from build123d import *

# Parameters (mm, degrees)
F0_W     = 31.75
F0_H     = 50.8
F0_W_2   = 3.175
F0_H_2   = 12.7
F0_W_3   = 12.7
F0_H_3   = 3.175
F0_W_4   = 19.05
F0_H_4   = 38.1
F1_DEPTH = 3.175


# Not quite as in the source:
# - a feature names something its author has since deleted; it is built from what else it names


with BuildPart() as f1:
    # F0 (on Top) → F1 (new body)
    with BuildSketch(Plane.XY):
        with Locations((-8.6727611423, -50.1471598029)):
            Rectangle(F0_W, F0_H)
        with Locations((-40.4227611423, -50.1471598029)):
            Rectangle(F0_W, F0_H)
        Polygon((-81.6977611423, 51.4528401971), (-88.0477611423, 51.4528401971), (-88.0477611423, 45.1028401971), (-84.8727611423, 45.1028401971), (-84.8727611423, 32.4028401971), (-84.8727611423, 19.7028401971), (-84.8727611423, 7.0028401971), (-84.8727611423, -5.6971598029), (-84.8727611423, -18.3971598029), (-88.0477611423, -18.3971598029), (-88.0477611423, -24.7471598029), (-68.9977611423, -24.7471598029), (-56.2977611423, -24.7471598029), (-24.5477611423, -24.7471598029), (7.2022388577, -24.7471598029), (19.9022388577, -24.7471598029), (38.9522388577, -24.7471598029), (38.9522388577, -18.3971598029), (35.7772388577, -18.3971598029), (35.7772388577, -5.6971598029), (35.7772388577, 7.0028401971), (35.7772388577, 19.7028401971), (35.7772388577, 32.4028401971), (35.7772388577, 45.1028401971), (38.9522388577, 45.1028401971), (38.9522388577, 51.4528401971), (32.6022388577, 51.4528401971), (32.6022388577, 48.2778401971), (19.9022388577, 48.2778401971), (7.2022388577, 48.2778401971), (-5.4977611423, 48.2778401971), (-18.1977611423, 48.2778401971), (-30.8977611423, 48.2778401971), (-43.5977611423, 48.2778401971), (-56.2977611423, 48.2778401971), (-68.9977611423, 48.2778401971), (-81.6977611423, 48.2778401971), align=None)
        with Locations((-86.4602611423, 26.0528401971)):
            Rectangle(F0_W_2, F0_H_2)
        with Locations((-86.4602611423, 0.6528401971)):
            Rectangle(F0_W_2, F0_H_2)
        with Locations((37.3647388577, 0.6528401971)):
            Rectangle(F0_W_2, F0_H_2)
        with Locations((37.3647388577, 26.0528401971)):
            Rectangle(F0_W_2, F0_H_2)
        with Locations((-62.6477611423, 49.8653401971)):
            Rectangle(F0_W_3, F0_H_3)
        with Locations((-11.8477611423, 49.8653401971)):
            Rectangle(F0_W_3, F0_H_3)
        with Locations((-37.2477611423, 49.8653401971)):
            Rectangle(F0_W_3, F0_H_3)
        with Locations((-78.5227611423, -43.7971598029)):
            Rectangle(F0_W_4, F0_H_4)
        with Locations((29.4272388577, -43.7971598029)):
            Rectangle(F0_W_4, F0_H_4)
        with Locations((13.5522388577, 49.8653401971)):
            Rectangle(F0_W_3, F0_H_3)
    extrude(amount=F1_DEPTH)


solid = f1.part
The model under review builds one solid part; all positions refer to its coordinate system, in mm. A direction names the side the tool comes from. Coordinates: 2 decimals unless noted, no trailing zeros. Write each loop counter-clockwise with the first axis right and the second up, starting at its lowest first coordinate (ties: lowest second). Pieces come first, ordered by that corner, then holes. Notation, with made-up numbers: (-3, 85) -> (4, 85) arc R27 cw to (4, 101) -> close; hole circle Ø6 at (-36, -1.75). An arc over 180 degrees is marked (long way). Answer in a Markdown table with one row per item.
1. For faces 4 (the flat face through (-63, -24.747, 2)), 5 (the flat face through (37, -5.697, 2)), 6 (the flat face through (-68.998, 50, 2)), list the 3-axis set-ups (+Z, -Z, +X, -X, +Y, -Y) from which the entire face can be reached by the end or side of a thin tool; tool diameter is ignored.
Answers below:
| item | result |
|---|---|
| face 4 | +Z, -Z, -Y |
| face 5 | +Z, -Z, +X |
| face 6 | +Z, -Z, +Y |
2. We need section A-A, the plane y = -56.5. State the section outline as (x, z) points (3 decimals), and give its area (3 significant figures).
Answers below:
| item | result |
|---|---|
| outline | (-88.048, 0) -> (-68.998, 0) -> (-68.998, 3.175) -> (-88.048, 3.175) -> close; (-56.298, 0) -> (7.202, 0) -> (7.202, 3.175) -> (-56.298, 3.175) -> close; (19.902, 0) -> (38.952, 0) -> (38.952, 3.175) -> (19.902, 3.175) -> close |
| area | 323 mm^2 |
3. We need section B-B, the plane x = 17. State the section outline as (y, z) points (3 decimals), and give its area (3 significant figures).
Answers below:
| item | result |
|---|---|
| outline | (-24.747, 0) -> (51.453, 0) -> (51.453, 3.175) -> (-24.747, 3.175) -> close |
| area | 242 mm^2 |
4. Draft analysis for pull direction X (two halves, no side actions). For faces 1 (the flat face through (-63, 51.453, 2)), 2 (the flat face through (-84.873, 39, 2)), 3 (the flat face through (19.902, -44, 2)), state which applies: +X half, -X half, draft (parallel to the pull), parting line (faces both ways), or undercut.
Answers below:
| item | result |
|---|---|
| face 1 | draft |
| face 2 | -X half |
| face 3 | undercut |
5. Clearance check with flat-ended pins moving along their axes: pin 1 Ø1 at (x, z) = (-23.5, 2) entering from +Y; pin 2 Ø1 at (x, z) = (37.5, 1.5) entering from -Y. State where each tip first meets the part, or that it passes through.
Answers below:
| item | result |
|---|---|
| pin 1 | stops at y = 48.28 |
| pin 2 | stops at y = -62.85 |
6. Wall thickness on probe 1 along X at (y, z) = (-59, 2.95); probe 2 along Y at (x, z) = (6.5, 0.35); probe 3 along X at (y, z) = (17, 3): over which ranges is each line inside the solid? List them lowest first. Write a range as [from, to].
Answers below:
| item | result |
|---|---|
| probe 1 | x = [-88.05, -69], [-56.3, 7.2], [19.9, 38.95] |
| probe 2 | y = [-75.55, 48.28] |
| probe 3 | x = [-84.87, 35.78] |
7. We need section C-C, the plane x = -49. State the section outline as (y, z) points (3 decimals).
Answers below:
| item | result |
|---|---|
| outline | (-75.547, 0) -> (48.278, 0) -> (48.278, 3.175) -> (-75.547, 3.175) -> close |
